The model under review builds one solid part; all positions refer to its coordinate system, in mm. Round coordinates to 2 decimals unless told otherwise and drop trailing zeros. Order: outer loops, then holes, each group sorted by start corner. A loop starts at its lowest first (then second) coordinate and runs counter-clockwise, first axis right, second up.
```python
from build123d import *

# Parameters (mm, degrees)
BOSS_EXTRUDE1_DEPTH                      = 3
MIRROR1_AT_THE_SECOND_PLANE_COPY_1_DEPTH = 3


with BuildPart() as part:
    # Sketch1 → Boss-Extrude1 (new body)
    with BuildSketch(Plane(origin=(0, 0, 0), x_dir=(1, 0, 0), z_dir=(0, 1, 0))):
        Polygon((-76, -76), (-59.111111111, -76), (-59.111111111, -73), (-42.222222222, -73), (-42.222222222, -76), (-25.333333333, -76), (-25.333333333, -73), (-8.444444444, -73), (-8.444444444, -76), (0, -76), (0, 0), (-76, 0), (-76, -8.444444444), (-73, -8.444444444), (-73, -25.333333333), (-76, -25.333333333), (-76, -42.222222222), (-73, -42.222222222), (-73, -59.111111111), (-76, -59.111111111), align=None)
    boss_extrude1 = extrude(amount=BOSS_EXTRUDE1_DEPTH)



with BuildPart() as mirror1_1:
    # Mirror1: Boss-Extrude1 across plane
    add(boss_extrude1.mirror(Plane.XY))


with BuildPart() as part_1:
    add(part.part)

    add(mirror1_1.part)  # Mirror1 at the second plane merges Mirror1_1
    # Mirror1 at the second plane: Boss-Extrude1 across plane
    add(boss_extrude1.mirror(Plane(origin=(0, 0, 0), x_dir=(0, 0, 1), z_dir=(1, 0, 0))))

    # Mirror1 at the second plane copy 1 sketc → Mirror1 at the second plane copy 1 (add)
    with BuildSketch(Plane(origin=(0, 0, 0), x_dir=(-1, 0, 0), z_dir=(0, 1, 0))):
        Polygon((-76, -76), (-59.111111111, -76), (-59.111111111, -73), (-42.222222222, -73), (-42.222222222, -76), (-25.333333333, -76), (-25.333333333, -73), (-8.444444444, -73), (-8.444444444, -76), (0, -76), (0, 0), (-76, 0), (-76, -8.444444444), (-73, -8.444444444), (-73, -25.333333333), (-76, -25.333333333), (-76, -42.222222222), (-73, -42.222222222), (-73, -59.111111111), (-76, -59.111111111), align=None)
    extrude(amount=MIRROR1_AT_THE_SECOND_PLANE_COPY_1_DEPTH)


solid = part_1.part
```
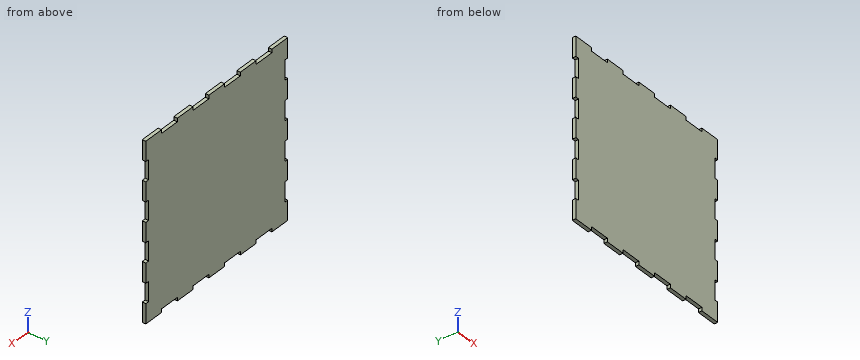
(1) Consider section A-A (z = 55). Write out the cut boundary in (x, y).
Data:
outline: (-73, 0) - (73, 0) - (73, 3) - (-73, 3) - close
(2) Consider section B-B (x = -23). Write out the cut boundary in (y, z).
Data:
outline: (0, -73) - (3, -73) - (3, 73) - (0, 73) - close
(3) Insertion check: pin 1 (1.5 mm diameter, centred on y = 1.5, z = -18.5, fed in from +X); pin 2 (1.5 mm diameter, centred on x = -49.5, y = 1, fed in from -Z). Each pin has a flat end and moves straight along its axis. Give the tip position at first contact, or say it passes through.
Data:
pin 1: stops at x = 73
pin 2: stops at z = -73
(4) To check wall thickness, follow probe 1 along X at (y, z) = (2.6, 25). State the ranges of the line that lie inside material, in increasing order.
Data:
probe 1: x = -73 to 73
